Here's how the part is built. I have some questions about the finished solid (model axes, mm). A direction names the side the tool comes from. Coordinates: 2 decimals unless noted, no trailing zeros. Write each loop counter-clockwise with the first axis right and the second up, starting at its lowest first coordinate (ties: lowest second). Pieces come first, ordered by that corner, then holes. Notation, with made-up numbers: (-17.75, 46.25) - (2.25, 46.25) arc R31 ccw to (2.25, 71.25) - close; hole circle Ø6 at (53, -23.5). An arc over 180 degrees is marked (long way). Answer in a Markdown table with one row per item. Add a question column.
Item 1: We'd pull the mould along Y, two halves only. Please class faces 3 (the face through (1.52, 19.39, -10.89)), 4 (the face through (1.52, 35.4, -23.43)), 5 (the face through (1.52, 0.57, -23.4)), 6 (the face through (23, 14, 3)): +Y half, -Y half, draft (parallel to the pull), parting line (faces both ways), or undercut.
Item 2: Which directions (+Z, -Z, +X, -X, +Y, -Y) give clear straight access to the entire face, cutting with the end or side of a thin tool? Please do faces 1 (the face through (10.5, 15.8, 1.5)), 2 (the face through (0, 18, -7)).
Item 3: I'm going to push flat-ended pins straight in: pin 1 (1 mm diameter, centred on x = 27.5, y = 5, fed in from -Z); pin 2 (2 mm diameter, centred on y = 18, z = -18, fed in from -X) (3 decimals). Where does each tip first touch, or does it pass through?
Item 4: If I drill on probe 1 along Y at (x, z) = (1.2, -10); probe 2 along X at (y, z) = (16.5, -8.5); probe 3 along Z at (x, y) = (10, 8.5), over which ranges is the centre line in solid material (lowest first)? Write a range as from..to.
Item 5: Imagine slicing it at A-A (z = -10). State how many separate pieces and enclosed holes the cut face has, plus the area to 3 significant figures.
Item 6: Imagine slicing it at B-B (y = 26). Please give me the cut outline in (x, z), plus the area to 3 significant figures.
Item 7: Imagine slicing it at C-C (x = 6). Please give me the cut outline in (y, z), plus the area to 3 significant figures.
from build123d import *

# Parameters (mm, degrees)
SKETCH_1_W          = 46
SKETCH_1_H          = 36
SKETCH_1_R          = 1.65
EXTRUDE_1_DEPTH     = 3
SKETCH_2_W          = 3
SKETCH_2_H          = 36
EXTRUDE_2_DEPTH     = 24
SKETCH_3_R          = 1.65
CUT_EXTRUDE_1_DEPTH = 50
FILLET_1_R          = 2


with BuildPart() as part:
    # 草图1 → 凸台-拉伸1 (new body)
    with BuildSketch(Plane.XY):
        with Locations((23, 18)):
            Rectangle(SKETCH_1_W, SKETCH_1_H)
        with BuildLine():
            Line((20.8, 30), (20.8, 31))
            ThreePointArc((20.8, 31), (23, 33.2), (25.2, 31))
            Line((25.2, 31), (25.2, 30))
            ThreePointArc((25.2, 30), (23, 27.8), (20.8, 30))
        make_face(mode=Mode.SUBTRACT)
        with BuildLine():
            ThreePointArc((36, 20.2), (38.2, 18), (36, 15.8))
            Line((36, 15.8), (35, 15.8))
            ThreePointArc((35, 15.8), (32.8, 18), (35, 20.2))
            Line((35, 20.2), (36, 20.2))
        make_face(mode=Mode.SUBTRACT)
        with BuildLine():
            ThreePointArc((25.2, 5), (23, 2.8), (20.8, 5))
            Line((20.8, 5), (20.8, 6))
            ThreePointArc((20.8, 6), (23, 8.2), (25.2, 6))
            Line((25.2, 6), (25.2, 5))
        make_face(mode=Mode.SUBTRACT)
        with BuildLine():
            ThreePointArc((10, 15.8), (7.8, 18), (10, 20.2))
            Line((10, 20.2), (11, 20.2))
            ThreePointArc((11, 20.2), (13.2, 18), (11, 15.8))
            Line((11, 15.8), (10, 15.8))
        make_face(mode=Mode.SUBTRACT)
        with Locations((23, 18)):
            Circle(SKETCH_1_R, mode=Mode.SUBTRACT)
    extrude(amount=EXTRUDE_1_DEPTH)

    # 草图2 → 凸台-拉伸2 (add)
    with BuildSketch(Plane.XY):
        with Locations((1.5, 18)):
            Rectangle(SKETCH_2_W, SKETCH_2_H)
        with Locations((44.5, 18)):
            Rectangle(SKETCH_2_W, SKETCH_2_H)
    extrude(amount=-EXTRUDE_2_DEPTH)

    # 草图3 → 切除-拉伸1 (cut)
    with BuildSketch(Plane(origin=(46, 0, 0), x_dir=(0, 0, -1), z_dir=(1, 0, 0))):
        with Locations((18, 10)):
            Circle(SKETCH_3_R)
        with Locations((10, 18)):
            Circle(SKETCH_3_R)
        with Locations((10, 10)):
            Circle(SKETCH_3_R)
        with Locations((18, 26)):
            Circle(SKETCH_3_R)
        with Locations((18, 18)):
            Circle(SKETCH_3_R)
        with Locations((10, 26)):
            Circle(SKETCH_3_R)
    extrude(amount=-CUT_EXTRUDE_1_DEPTH, mode=Mode.SUBTRACT)

    # 圆角1
    fillet_1_edges = [part.edges().sort_by_distance(p)[0] for p in [
        (1.5, 36, -24),
        (1.5, 0, -24),
        (44.5, 0, -24),
        (44.5, 36, -24),
    ]]
    fillet(fillet_1_edges, radius=FILLET_1_R)


solid = part.part
Here are the results:
| question | item | result |
|---|---|---|
| 1 | face 3 | undercut |
| 1 | face 4 | +Y half |
| 1 | face 5 | -Y half |
| 1 | face 6 | draft |
| 2 | face 1 | +Z, -Z |
| 2 | face 2 | +Z, -Z, -X, +Y, -Y |
| 3 | pin 1 | stops at z = 0 |
| 3 | pin 2 | passes through |
| 4 | probe 1 | y = 0..8.35, 11.65..16.35, 19.65..24.35, 27.65..36 |
| 4 | probe 2 | x = 0..3, 43..46 |
| 4 | probe 3 | z = 0..3 |
| 5 | separate pieces | 8 |
| 5 | enclosed holes | 0 |
| 5 | area | 157 mm2 |
| 6 | outline | (0, -24) - (3, -24) - (3, -19.65) - (0, -19.65) - close; (0, -16.35) - (3, -16.35) - (3, -11.65) - (0, -11.65) - close; (0, -8.35) - (3, -8.35) - (3, 0) - (43, 0) - (43, -8.35) - (46, -8.35) - (46, 3) - (0, 3) - close; (43, -24) - (46, -24) - (46, -19.65) - (43, -19.65) - close; (43, -16.35) - (46, -16.35) - (46, -11.65) - (43, -11.65) - close |
| 6 | area | 242 mm2 |
| 7 | outline | (0, 0) - (36, 0) - (36, 3) - (0, 3) - close |
| 7 | area | 108 mm2 |
